```python
from build123d import *

# Parameters (mm, degrees)
SKETCH_1_W          = 20
SKETCH_1_H          = 20
EXTRUDE_1_DEPTH     = 10
SKETCH_2_R          = 5
CUT_EXTRUDE_2_DEPTH = 18.320508076
SKETCH_3_W          = 5
SKETCH_3_H          = 20
EXTRUDE_2_DEPTH     = 20
SKETCH_4_R          = 5
CUT_EXTRUDE_3_DEPTH = 31


with BuildPart() as part:
    # 草图1 → 凸台-拉伸1 (new body)
    with BuildSketch(Plane(origin=(0, 0, 0), x_dir=(1, 0, 0), z_dir=(0, 1, 0))):
        Rectangle(SKETCH_1_W, SKETCH_1_H)
    extrude(amount=EXTRUDE_1_DEPTH)

    # 草图2 → 切除-拉伸2 (cut, through all)
    with BuildSketch(Plane(origin=(0, 10, 0), x_dir=(1, 0, 0), z_dir=(0, 1, 0))):
        with Locations(Location((0, 0, 0), (0, 0, 270))):
            Circle(SKETCH_2_R)
    extrude(amount=-CUT_EXTRUDE_2_DEPTH, mode=Mode.SUBTRACT)

    # 草图3 → 凸台-拉伸2 (add)
    with BuildSketch(Plane.XZ):
        with Locations((-7.5, 0)):
            Rectangle(SKETCH_3_W, SKETCH_3_H)
        with Locations((7.5, 0)):
            Rectangle(SKETCH_3_W, SKETCH_3_H)
    extrude(amount=EXTRUDE_2_DEPTH)

    # 草图4 → 切除-拉伸3 (cut, through all)
    with BuildSketch(Plane.ZY.offset(10)):
        with Locations((0, -10)):
            Circle(SKETCH_4_R)
    extrude(amount=-CUT_EXTRUDE_3_DEPTH, mode=Mode.SUBTRACT)


solid = part.part
```
Work out the finished part from the listing and answer in its coordinate system (mm). A direction names the side the tool comes from. Give positions to 0.01 mm unless a question says otherwise; leave off trailing zeros. Write each loop counter-clockwise with the first axis right and the second up, starting at its lowest first coordinate (ties: lowest second). Pieces come first, ordered by that corner, then holes.
(1) The part is cut by section D-D on y = 4.5. Write down the section's boundary in (x, z).
Final values:
outline: (-10, -10) - (10, -10) - (10, 10) - (-10, 10) - close; hole circle Ø10 at (0, 0)
(2) Straight lines are drawn through the part: line 1 (X direction, y = 6.5, z = 0); line 2 (Y direction, x = -7.05, z = 0); line 3 (Y direction, x = 0, z = 8). For each, find the intervals that lie inside material, in ascending order.
Final values:
line 1: x = -10 to -5, 5 to 10
line 2: y = -20 to -15, -5 to 10
line 3: y = 0 to 10
(3) Which of the six approach directions +Z, -Z, +X, -X, +Y, -Y give full straight-line access (tool end or side, diameter ignored) to faces 1 (the flat face through (0, 2, -10)), 2 (the flat face through (0, 0, 7))?
Final values:
face 1: -Z, +X, -X, +Y, -Y
face 2: +Z, -Z, -Y
(4) The mould has two halves that part along X. Classify faces 3 (the flat face through (0, 0, -7)), 4 (the cylindrical face through (7.465, -5.043, -0.651)), 5 (the flat face through (-10, -4.8, -0.1)): pulls with the +X half, pulls with the -X half, needs draft (parallel to the pull), parting line crosses it, or undercut.
Final values:
face 3: undercut
face 4: needs draft
face 5: pulls with the -X half
(5) The part is cut by section B-B on x = 6.5. Write down the section's boundary in (y, z).
Final values:
outline: (-20, -10) - (10, -10) - (10, 10) - (-20, 10) - close; hole circle Ø10 at (-10, 0)
(6) The part is cut by section A-A on y = -1.5. Write down the section's boundary in (x, z).
Final values:
outline: (-10, -10) - (-5, -10) - (-5, 10) - (-10, 10) - close; (5, -10) - (10, -10) - (10, 10) - (5, 10) - close
(7) The part is cut by section C-C on z = 5.5. Write down the section's boundary in (x, y).
Final values:
outline: (-10, -20) - (-5, -20) - (-5, 0) - (5, 0) - (5, -20) - (10, -20) - (10, 10) - (-10, 10) - close
(8) A flat-ended cylindrical pin translates along its axis: pin 1 Ø3 at (x, z) = (-1, 6) entering from -Y. Find the tip coordinate at first contact, or state that the pin passes through.
Final values:
pin 1: stops at y = 0
